Autodesk Inventor part; units mm, degrees
ref_plane "bp_b_oben_XY" through (30, 0, -5) normal (0, 1, 0) x (1, 0, 0)
ref_plane "bp_b_oben_YZ" through (30, 0, -5) normal (1, 0, 0) x (0, 0, -1)
ref_plane "bp_b_oben_ZX" through (30, 0, -5) normal (0, 0, -1) x (0, 1, 0)
sketch "Sketch_1" plane through (0, 0, 0) normal (0, 1, 0) x (-1, 0, 0)
  arc A0 (35, 0) -> (30, 5) centre (30, 0) ccw
  line L0 (30, 5) -> (-30, 5)
  arc A1 (-30, 5) -> (-35, 0) centre (-30, 0) ccw
  arc A2 (-35, 0) -> (-30, -5) centre (-30, 0) ccw
  line L1 (-30, -5) -> (30, -5)
  arc A3 (30, -5) -> (35, 0) centre (30, 0) ccw
extrude "Extrusion1" add sketch "Sketch_1" along normal mid plane 8
ref_plane "bp_b_oben_XY" through (30, 0, -5) normal (0, 1, 0) x (1, 0, 0)
ref_plane "bp_b_oben_YZ" through (30, 0, -5) normal (1, 0, 0) x (0, 0, -1)
ref_plane "bp_b_oben_ZX" through (30, 0, -5) normal (0, 0, -1) x (0, 1, 0)
ref_plane "bp_b_unten_XY" through (30, 0, 5) normal (0, 1, 0) x (1, 0, 0)
ref_plane "bp_b_unten_YZ" through (30, 0, 5) normal (1, 0, 0) x (0, 0, -1)
ref_plane "bp_b_unten_ZX" through (30, 0, 5) normal (0, 0, -1) x (0, 1, 0)
ref_plane "bp_h_oben_XY" through (0, 4, 0) normal (0, 0, 1) x (1, 0, 0)
ref_plane "bp_h_oben_YZ" through (0, 4, 0) normal (1, 0, 0) x (0, 1, 0)
ref_plane "bp_h_oben_ZX" through (0, 4, 0) normal (0, 1, 0) x (0, 0, 1)
ref_plane "bp_h_unten_XY" through (0, -4, 0) normal (0, 0, 1) x (1, 0, 0)
ref_plane "bp_h_unten_YZ" through (0, -4, 0) normal (1, 0, 0) x (0, 1, 0)
ref_plane "bp_h_unten_ZX" through (0, -4, 0) normal (0, 1, 0) x (0, 0, 1)
ref_plane "bp_l_links_XY" through (-35, 0, 0) normal (0, 1, 0) x (1, 0, 0)
ref_plane "bp_l_links_YZ" through (-35, 0, 0) normal (1, 0, 0) x (0, 0, -1)
ref_plane "bp_l_links_ZX" through (-35, 0, 0) normal (0, 0, -1) x (0, 1, 0)
ref_plane "bp_l_rechts_XY" through (35, 0, 0) normal (0, 1, 0) x (1, 0, 0)
ref_plane "bp_l_rechts_YZ" through (35, 0, 0) normal (1, 0, 0) x (0, 0, -1)
ref_plane "bp_l_rechts_ZX" through (35, 0, 0) normal (0, 0, -1) x (0, 1, 0)
properties part number "K0696.110X70"
Geometry check sheet. Reference: the model listing, model coordinates, mm. Give positions to 0.01 mm unless a question says otherwise; leave off trailing zeros. Write each loop counter-clockwise with the first axis right and the second up, starting at its lowest first coordinate (ties: lowest second). Pieces come first, ordered by that corner, then holes.
1) Section check B-B, the plane y = 2.25. Record the boundary of the cut face in (x, z).
2) Section check A-A, the plane z = -3. Record the boundary of the cut face in (x, y), and give its area (3 significant figures).
3) Material ranges on L1, parallel to Z at x = 30.5, y = 3.25; L2, parallel to X at y = -1, z = 0.5; L3, parallel to X at y = -1, z = -4, recorded low to high.
Computed:
1. outline: (-30, -5) - (30, -5) arc R5 ccw to (30, 5) - (-30, 5) arc R5 ccw to start
2. outline: (-34, -4) - (34, -4) - (34, 4) - (-34, 4) - close
2. area: 544 mm2
3. L1: z = -4.97 to 4.97
3. L2: x = -34.97 to 34.97
3. L3: x = -33 to 33
